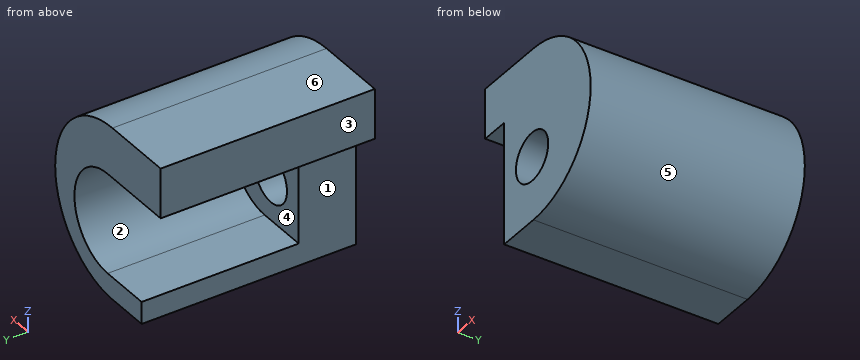
```python
from build123d import *

# Parameters (mm, degrees)
SKETCH1_R           = 1.7
BOSS_EXTRUDE2_DEPTH = 4
BOSS_EXTRUDE3_DEPTH = 15


with BuildPart() as part:
    # Sketch1 → Boss-Extrude2 (new body)
    with BuildSketch(Plane(origin=(0, 0, 0), x_dir=(1, 0, 0), z_dir=(0, 1, 0))):
        with BuildLine():
            Line((-2.93579488, -0.53336368), (-2.93579488, 2.96663632))
            Line((-2.93579488, 2.96663632), (0.643666224, 2.96663632))
            ThreePointArc((0.643666224, 2.96663632), (4.143666224, -0.53336368), (0.643666224, -4.03336368))
            Line((0.643666224, -4.03336368), (-2.93579488, -4.03336368))
            Line((-2.93579488, -4.03336368), (-2.93579488, -0.53336368))
        make_face()
        with Locations(Location((0, 0, 0), (0, 0, 270))):
            Circle(SKETCH1_R, mode=Mode.SUBTRACT)
    extrude(amount=BOSS_EXTRUDE2_DEPTH)

    # Sketch2 → Boss-Extrude3 (add)
    with BuildSketch(Plane(origin=(0, 0, 0), x_dir=(1, 0, 0), z_dir=(0, 1, 0))):
        with BuildLine():
            Line((-2.93579488, 4.517571778), (0.143666226, 4.517571778))
            ThreePointArc((0.143666226, 4.517571778), (6.169133955, -1.507895951), (0.143666226, -7.53336368))
            Line((0.143666226, -7.53336368), (-3.435794878, -7.53336368))
            Line((-3.435794878, -7.53336368), (-4.93579488, -7.53336368))
            Line((-4.93579488, -7.53336368), (-4.93579488, -4.03336368))
            Line((-4.93579488, -4.03336368), (-2.93579488, -4.03336368))
            Line((-2.93579488, -4.03336368), (0.643666224, -4.03336368))
            ThreePointArc((0.643666224, -4.03336368), (4.143666224, -0.53336368), (0.643666224, 2.96663632))
            Line((0.643666224, 2.96663632), (-2.93579488, 2.96663632))
            Line((-2.93579488, 2.96663632), (-2.93579488, 4.517571778))
        make_face()
    extrude(amount=BOSS_EXTRUDE3_DEPTH)


solid = part.part
```
Read the model definition and answer for the solid it produces. Units are mm, in the model's axes. Face numbers are marked on the shaded views. A direction names the side the tool comes from. Coordinates: 2 decimals unless noted, no trailing zeros. Write each loop counter-clockwise with the first axis right and the second up, starting at its lowest first coordinate (ties: lowest second). Pieces come first, ordered by that corner, then holes. Notation, with made-up numbers: (-26.75, 41) -> (-2.75, 41) arc R17 ccw to (-2.75, 52) -> close; hole circle Ø1 at (-35, 8). An arc over 180 degrees is marked (long way). Write item = value, one per line.
(1) Section B-B on x = -2.75 is taken. Write down the section's boundary in (y, z), plus the area to 3 significant figures.
From the geometry:
outline = (0, -4.52) -> (15, -4.52) -> (15, -2.97) -> (4, -2.97) -> (4, 4.03) -> (15, 4.03) -> (15, 7.53) -> (0, 7.53) -> close
area = 104 mm2
(2) Which of the six approach directions +Z, -Z, +X, -X, +Y, -Y give full straight-line access (tool end or side, diameter ignored) to the marked faces 1, 2 and 3?
From the geometry:
face_1 = -Z, -X, +Y, -Y
face_2 = -X, +Y
face_3 = +Z, -Z, -X, +Y, -Y
(3) Section D-D on z = 0 is taken. Write down the section's boundary in (x, y).
From the geometry:
outline = (-2.94, 0) -> (-1.7, 0) -> (-1.7, 4) -> (-2.94, 4) -> close; (1.7, 0) -> (5.98, 0) -> (5.98, 15) -> (4.1, 15) -> (4.1, 4) -> (1.7, 4) -> close
(4) Straight lines are drawn through the part: L1, parallel to Z at x = -0.5, y = 12; L2, parallel to X at y = 1.6, z = 0; L3, parallel to Y at x = -2.25, z = -1.25. For each, find the intervals that lie inside material, in ascending order. Write a range as from..to.
From the geometry:
L1 = -4.52..-2.97, 4.03..7.53
L2 = -2.94..-1.7, 1.7..5.98
L3 = 0..4
(5) For a pull along Z with two mould halves and no side action, classify the marked faces 4, 5 and 6 as +Z half, -Z half, draft (parallel to the pull), parting line (faces both ways), or undercut.
From the geometry:
face_4 = undercut
face_5 = parting line
face_6 = +Z half
(6) Given pin 1 Ø4.5 at (y, z) = (4, -0.5) entering from -X; pin 2 Ø2 at (y, z) = (6.5, -0.5) entering from -X; pin 3 Ø1.5 at (y, z) = (7.5, -2.5) entering from +X, each flat-ended and moving along its own axis, determine where each tip first touches the part or whether it passes through.
From the geometry:
pin_1 = -2.94
pin_2 = 3.49
pin_3 = 5.21
